The model under review builds one solid part; all positions refer to its coordinate system, in mm. A direction names the side the tool comes from. Give positions to 0.01 mm unless a question says otherwise; leave off trailing zeros. Order: outer loops, then holes, each group sorted by start corner. A loop starts at its lowest first (then second) coordinate and runs counter-clockwise, first axis right, second up. Notation, with made-up numbers: (5, -37.75) - (34, -37.75) arc R14 ccw to (34, -17.75) - close; hole circle Ø5 at (-19, 88.5). An arc over 180 degrees is marked (long way). Put each result on its own line as item: value.
```python
from build123d import *

# Parameters (mm, degrees)
SKETCH1_R                                 = 13.45
PISTON_DEPTH                              = 5
SKETCH2_R                                 = 6.35
ROD_DEPTH                                 = 20.153
F_106_5_16_24_INTERNAL_THREAD_D           = 6.9088
F_106_5_16_24_INTERNAL_THREAD_DEPTH       = 16.37754
F_106_5_16_24_INTERNAL_THREAD_CBORE_D     = 7.9375
F_106_5_16_24_INTERNAL_THREAD_CBORE_DEPTH = 13.208
F_106_5_16_24_INTERNAL_THREAD_TIP         = 2.075612922
ROD_END_CHAMFER_SIZE                      = 1
WRENCH_FLATS_DEPTH                        = 28.711882091
WRENCH_FLATS_DEPTH_BACK                   = 28.711882091


with BuildPart() as part:
    # Sketch1 → Piston (new body)
    with BuildSketch(Plane.XY):
        Circle(SKETCH1_R)
    extrude(amount=PISTON_DEPTH)

    # Sketch2 → Rod (add)
    with BuildSketch(Plane(origin=(0, 0, 0), x_dir=(-1, 0, 0), z_dir=(0, 0, -1))):
        with Locations(Location((0, 0, 0), (0, 0, 90))):
            Circle(SKETCH2_R)
    extrude(amount=-ROD_DEPTH)

    # 106 5/16-24 Internal Thread
    with Locations(Plane(origin=(0, 0, 20.153), x_dir=(0, 1, 0), z_dir=(0, 0, 1))):
        with Locations((0, 0)):
            CounterBoreHole(F_106_5_16_24_INTERNAL_THREAD_D / 2, F_106_5_16_24_INTERNAL_THREAD_CBORE_D / 2, F_106_5_16_24_INTERNAL_THREAD_CBORE_DEPTH, depth=F_106_5_16_24_INTERNAL_THREAD_DEPTH)
            with Locations((0, 0, -(F_106_5_16_24_INTERNAL_THREAD_DEPTH + F_106_5_16_24_INTERNAL_THREAD_TIP / 2))):  # 118° drill point
                Cone(0, F_106_5_16_24_INTERNAL_THREAD_D / 2, F_106_5_16_24_INTERNAL_THREAD_TIP, mode=Mode.SUBTRACT)

    # Rod End Chamfer
    rod_end_chamfer_edges = [part.edges().sort_by_distance(p)[0] for p in [
        (0, -3.96875, 20.153),
        (0, -6.35, 20.153),
    ]]
    chamfer(rod_end_chamfer_edges, length=ROD_END_CHAMFER_SIZE)

    # Sketch11 → Wrench Flats (cut, two sides: drawn at the far end of the back side and taken through both)
    with BuildSketch(Plane(origin=(0, 0, 0), x_dir=(1, 0, 0), z_dir=(0, 1, 0)).offset(-WRENCH_FLATS_DEPTH_BACK)):
        Polygon((-5.55, -20.153), (-5.55, -17.153), (-10.55, -14.266248654), (-10.55, -20.153), align=None)
        Polygon((5.55, -20.153), (5.55, -17.153), (10.55, -14.266248654), (10.55, -20.153), align=None)
    extrude(amount=WRENCH_FLATS_DEPTH + WRENCH_FLATS_DEPTH_BACK, mode=Mode.SUBTRACT)


solid = part.part
```
(1) Wall thickness on L1, parallel to X at y = 0, z = 5.8; L2, parallel to Z at x = -11, y = 2; L3, parallel to X at y = 0, z = 15: over which ranges is each line inside the solid? List them lowest first.
The answers:
L1: -6.35 to -3.45, 3.45 to 6.35
L2: 0 to 5
L3: -6.35 to -3.97, 3.97 to 6.35
(2) For faces 4 (the flat face through (5.55, 0, 19)), 5 (the flat face through (-5.55, 0, 19)), 6 (the cylindrical face through (3.874, -0.86, 13.134)), list the 3-axis set-ups (+Z, -Z, +X, -X, +Y, -Y) from which the entire face can be reached by the end or side of a thin tool; tool diameter is ignored.
The answers:
face 4: +Z, +X, +Y, -Y
face 5: +Z, -X, +Y, -Y
face 6: +Z
(3) Take a section at B-B, the plane x = 9.25. Write out the cut boundary in (y, z).
The answers:
outline: (-9.76, 0) - (9.76, 0) - (9.76, 5) - (-9.76, 5) - close
(4) Take a section at A-A, the plane z = 5.5. Write out the cut boundary in (x, y), then the cut area to 3 significant figures.
The answers:
outline: circle Ø12.7 at (0, 0); hole circle Ø6.91 at (0, 0)
area: 89.2 mm^2
(5) Take a section at C-C, the plane y = -8.5. Write out the cut boundary in (x, z), then the cut area to 3 significant figures.
The answers:
outline: (-10.42, 0) - (10.42, 0) - (10.42, 5) - (-10.42, 5) - close
area: 104 mm^2
(6) Clearance check with flat-ended pins moving along their axes: pin 1 Ø10 at (x, z) = (7, 5.5) entering from -Y; pin 2 Ø8 at (x, y) = (-10, 5.5) entering from +Z; pin 3 Ø1 at (x, y) = (3.5, 8) entering from -Z; pin 4 Ø6.5 at (x, y) = (0, 0) entering from +Z. State where each tip first meets the part, or that it passes through.
The answers:
pin 1: y = -13.3
pin 2: z = 5
pin 3: z = 0
pin 4: z = 3.65
(7) The part is to be moulded in two halves that separate along X. For faces 1 (the flat face through (0, 0, 0)), 2 (the conical face through (0.53, 0.28, 2.06)), 3 (the cylindrical face through (6.3, -0.8, 12)), say which applies: pulls with the +X half, pulls with the -X half, needs draft (parallel to the pull), parting line crosses it, or undercut.
The answers:
face 1: needs draft
face 2: undercut
face 3: parting line crosses it
